Here's how the part is built. I have some questions about the finished solid (model axes, mm). A direction names the side the tool comes from. Coordinates: 2 decimals unless noted, no trailing zeros. Loops run counter-clockwise (first coordinate to the right, second up) from the corner with the lowest first, then second, coordinate; pieces in that order, holes last. Notation, with made-up numbers: (84.5, -5.5) -> (110.5, -5.5) arc R24 ccw to (110.5, 25.5) -> close; hole circle Ø1 at (56, 81.25). An arc over 180 degrees is marked (long way). Answer as a JSON object with one key per item and string values. Group by question number.
1) I need wall thicknesses on probe 1 along X at (y, z) = (-32.5, 6.5); probe 2 along Y at (x, z) = (1.5, 5); probe 3 along Y at (x, z) = (-32, 2.5). Which ranges of each line are inside material? Lowest first, please. Write a range as [from, to].
2) I want a section at C-C (y = -82). Write out the boundary of the cut face in (x, z), then the cut area to 3 significant figures.
3) I want a section at A-A (x = 1). Write out the boundary of the cut face in (y, z), then the cut area to 3 significant figures.
4) Which directions (+Z, -Z, +X, -X, +Y, -Y) give clear straight access to the entire face, cutting with the end or side of a thin tool? Please do faces 5 (the flat face through (42.818, -36, 9)), 6 (the flat face through (0, -103.086, 5)), 7 (the flat face through (-16.182, 37, 4)).
5) I want a section at B-B (z = 2.25). Count the separate pieces of the cut face and the enclosed holes in it, then the cut area to 3 significant figures.
6) If we mould it in two halves opening along X, with no side actions, what happens to faces 1 (the cylindrical face through (50.62, 55.77, 4.93)), 2 (the cylindrical face through (-13.57, 46.76, 8.52)), 3 (the flat face through (0, -94.086, 9)), 4 (the flat face through (-1, 56.914, 5))? For each: +X half, -X half, draft (parallel to the pull), parting line (faces both ways), or undercut.
7) I'm going to push flat-ended pins straight in: pin 1 (1 mm diameter, centred on x = 12.5, y = -20.5, fed in from +Z); pin 2 (8 mm diameter, centred on x = 30.82, y = 38.91, fed in from -Z). Where does each tip first touch, or does it pass through?
8) I want a section at D-D (x = -25). Write out the boundary of the cut face in (y, z), then the cut area to 3 significant figures.
```python
from build123d import *

# Parameters (mm, degrees)
BOSS_EXTRUDE1_DEPTH = 10
CUT_EXTRUDE1_DEPTH  = 3
SKETCH4_W           = 30
SKETCH4_H           = 10
SKETCH4_W_2         = 25
SKETCH4_H_2         = 70
CUT_EXTRUDE3_DEPTH  = 7
SKETCH5_R           = 5
CUT_EXTRUDE4_DEPTH  = 10


with BuildPart() as part:
    # Sketch1 → Boss-Extrude1 (new body)
    with BuildSketch(Plane.XY):
        with BuildLine():
            Line((-49.181793273, 56.913856582), (47.818206727, 56.913856582))
            ThreePointArc((47.818206727, 56.913856582), (50.646633852, 55.742283706), (51.818206727, 52.913856582))
            Line((51.818206727, 52.913856582), (51.818206727, -99.086143418))
            ThreePointArc((51.818206727, -99.086143418), (50.646633852, -101.914570543), (47.818206727, -103.086143418))
            Line((47.818206727, -103.086143418), (-49.181793273, -103.086143418))
            ThreePointArc((-49.181793273, -103.086143418), (-52.010220398, -101.914570543), (-53.181793273, -99.086143418))
            Line((-53.181793273, -99.086143418), (-53.181793273, 52.913856582))
            ThreePointArc((-53.181793273, 52.913856582), (-52.010220398, 55.742283706), (-49.181793273, 56.913856582))
        make_face()
    extrude(amount=BOSS_EXTRUDE1_DEPTH)

    # Sketch3 → Cut-Extrude1 (cut)
    with BuildSketch(Plane.XY.offset(10)):
        with BuildLine():
            Line((-9.432728483, 47.913856582), (8.069141937, 47.913856582))
            ThreePointArc((8.069141937, 47.913856582), (12.15285738, 46.793047536), (15.09230652, 43.744673627))
            Line((15.09230652, 43.744673627), (41.84137131, -5.295278488))
            ThreePointArc((41.84137131, -5.295278488), (42.570152182, -7.149395843), (42.818206727, -9.126095533))
            Line((42.818206727, -9.126095533), (42.818206727, -64.086143418))
            ThreePointArc((42.818206727, -64.086143418), (34.031410163, -85.299346854), (12.818206727, -94.086143418))
            Line((12.818206727, -94.086143418), (-14.181793273, -94.086143418))
            ThreePointArc((-14.181793273, -94.086143418), (-35.394996709, -85.299346854), (-44.181793273, -64.086143418))
            Line((-44.181793273, -64.086143418), (-44.181793273, -9.126095533))
            ThreePointArc((-44.181793273, -9.126095533), (-43.933738728, -7.149395843), (-43.204957856, -5.295278488))
            Line((-43.204957856, -5.295278488), (-16.455893066, 43.744673627))
            ThreePointArc((-16.455893066, 43.744673627), (-13.516443926, 46.793047536), (-9.432728483, 47.913856582))
        make_face()
    extrude(amount=-CUT_EXTRUDE1_DEPTH, mode=Mode.SUBTRACT)

    # Sketch4 → Cut-Extrude3 (cut)
    with BuildSketch(Plane.XY.offset(7)):
        with Locations((-1.181793273, 36.913856582)):
            Rectangle(SKETCH4_W, SKETCH4_H)
        with Locations((-1.181793273, 11.913856582)):
            Rectangle(SKETCH4_W, SKETCH4_H)
        with Locations((-28.681793273, -28.086143418)):
            Rectangle(SKETCH4_W_2, SKETCH4_H)
        with Locations((27.318206727, -28.086143418)):
            Rectangle(SKETCH4_W_2, SKETCH4_H)
        with Locations((-0.681793273, -50.086143418)):
            Rectangle(SKETCH4_W_2, SKETCH4_H_2)
    extrude(amount=-CUT_EXTRUDE3_DEPTH, mode=Mode.SUBTRACT)

    # Sketch5 → Cut-Extrude4 (cut)
    with BuildSketch(Plane.XY.offset(10)):
        with Locations((30.818206727, 38.913856582)):
            Circle(SKETCH5_R)
    extrude(amount=-CUT_EXTRUDE4_DEPTH, mode=Mode.SUBTRACT)


solid = part.part
```
Determined:
{
 "1": {"probe 1": "[-53.18, -41.18], [-16.18, -13.18], [11.82, 14.82], [39.82, 51.82]", "probe 2": "[-103.09, -85.09], [-15.09, 6.91], [16.91, 31.91], [41.91, 56.91]", "probe 3": "[-103.09, -33.09], [-23.09, 56.91]"},
 "2": {"outline": "(-53.18, 0) -> (-13.18, 0) -> (-13.18, 7) -> (-38.25, 7) -> (-38.25, 10) -> (-53.18, 10) -> close; (11.82, 0) -> (51.82, 0) -> (51.82, 10) -> (36.88, 10) -> (36.88, 7) -> (11.82, 7) -> close", "area": "650 mm^2"},
 "3": {"outline": "(-103.09, 0) -> (-85.09, 0) -> (-85.09, 7) -> (-94.09, 7) -> (-94.09, 10) -> (-103.09, 10) -> close; (-15.09, 0) -> (6.91, 0) -> (6.91, 7) -> (-15.09, 7) -> close; (16.91, 0) -> (31.91, 0) -> (31.91, 7) -> (16.91, 7) -> close; (41.91, 0) -> (56.91, 0) -> (56.91, 10) -> (47.91, 10) -> (47.91, 7) -> (41.91, 7) -> close", "area": "544 mm^2"},
 "4": {"face 5": "+Z", "face 6": "+Z, -Z, +X, -X, -Y", "face 7": "+Z, -Z"},
 "5": {"separate pieces": "1", "enclosed holes": "6", "area": "13,900 mm^2"},
 "6": {"face 1": "+X half", "face 2": "undercut", "face 3": "undercut", "face 4": "draft"},
 "7": {"pin 1": "z = 7", "pin 2": "through"},
 "8": {"outline": "(-103.09, 0) -> (-33.09, 0) -> (-33.09, 7) -> (-92.07, 7) -> (-92.07, 10) -> (-103.09, 10) -> close; (-23.09, 0) -> (56.91, 0) -> (56.91, 10) -> (28.08, 10) -> (28.08, 7) -> (-23.09, 7) -> close", "area": "1,170 mm^2"}
}
